```python
from build123d import *

# Parameters (mm, degrees)
SKETCH1_W           = 66.15
SKETCH1_H           = 4
SKETCH1_H_2         = 29.25
SKETCH1_R           = 1.5
BOSS_EXTRUDE1_DEPTH = 4
BOSS_EXTRUDE2_START = 4
SKETCH1_3_W         = 66.15
SKETCH1_3_H         = 4
BOSS_EXTRUDE2_DEPTH = 9
SKETCH2_R           = 1.5
SKETCH2_R_2         = 2.031128953
CUT_EXTRUDE1_DEPTH  = 9


with BuildPart() as part:
    # Sketch1 → Boss-Extrude1 (new body)
    with BuildSketch(Plane(origin=(0, 0, 0), x_dir=(1, 0, 0), z_dir=(0, 1, 0))):
        with Locations((0, -16.625)):
            Rectangle(SKETCH1_W, SKETCH1_H)
        Rectangle(SKETCH1_W, SKETCH1_H_2)
        with Locations((28.075, 9.625)):
            Circle(SKETCH1_R, mode=Mode.SUBTRACT)
        with Locations((28.075, -9.625)):
            Circle(SKETCH1_R, mode=Mode.SUBTRACT)
        with Locations((-28.075, -9.625)):
            Circle(SKETCH1_R, mode=Mode.SUBTRACT)
        with Locations((-28.075, 9.625)):
            Circle(SKETCH1_R, mode=Mode.SUBTRACT)
    extrude(amount=BOSS_EXTRUDE1_DEPTH)

    # Sketch1<3> → Boss-Extrude2 (add)
    with BuildSketch(Plane(origin=(0, 0, 0), x_dir=(1, 0, 0), z_dir=(0, 1, 0)).offset(BOSS_EXTRUDE2_START)):
        with Locations((0, -16.625)):
            Rectangle(SKETCH1_3_W, SKETCH1_3_H)
    extrude(amount=BOSS_EXTRUDE2_DEPTH)

    # Sketch2 → Cut-Extrude1 (cut)
    with BuildSketch(Plane.XY.offset(18.625)):
        with Locations((-24.96, 9)):
            Circle(SKETCH2_R)
        with Locations((24.96, 9)):
            Circle(SKETCH2_R_2)
    extrude(amount=-CUT_EXTRUDE1_DEPTH, mode=Mode.SUBTRACT)


solid = part.part
```
Check sheet for the modelled part. Datum: model origin and axes. Units: mm. A direction names the side the tool comes from. Give positions to 0.01 mm unless a question says otherwise; leave off trailing zeros. Order: outer loops, then holes, each group sorted by start corner. A loop starts at its lowest first (then second) coordinate and runs counter-clockwise, first axis right, second up. Notation, with made-up numbers: (-5.75, 51.5) -> (23.25, 51.5) arc R9 ccw to (23.25, 67.5) -> close; hole circle Ø7 at (71.5, 33). An arc over 180 degrees is marked (long way). Use CSV: the item, a comma, the result in double quotes. Start each with the question number.
1) Material ranges on line 1 (X direction, y = 1.75, z = 11) (3 decimals); line 2 (X direction, y = 1.75, z = -10) (3 decimals); line 3 (Y direction, x = -24.96, z = 17.15), recorded low to high. Write a range as from..to.
2) Set-up check for faces 1 (the face through (0, 8, 14.625)), 2 (the face through (0, 6, 18.625)): record each of +Z, -Z, +X, -X, +Y, -Y from which the full face is reachable in a straight line by a thin tool's end or side.
3) Sectioned sample at A-A, the plane x = 24.96. Record the boundary of the cut face in (y, z) (3 decimals), plus the area to 3 significant figures.
4) Mould release check, pull along Y, two halves, no side actions. Record for faces 3 (the face through (-26.69, 1.97, 10.2)), 4 (the face through (23.46, 10.37, 16.65)), 5 (the face through (0, 0, 2)), 6 (the face through (0, 4, 0)): released by +Y, released by -Y, zero draft, split by the parting line, or undercut.
5) Sectioned sample at C-C, the plane z = -9. Record the boundary of the cut face in (x, y) (3 decimals), plus the area to 3 significant figures.
6) Go/stop test with flat-tipped pins: P1, Ø3, axis at x = -19, z = 7.5, coming from the +Y side; P2, Ø5, axis at y = 8, z = 11, coming from the +X side; P3, Ø2.5, axis at x = -16, y = 7, coming from the -Z side (3 decimals). Record where each tip stops, or that it passes through.
7) Sectioned sample at B-B, the plane y = 9. Record the boundary of the cut face in (x, z) (3 decimals).
8) Sectioned sample at D-D, the plane x = -24.96. Record the boundary of the cut face in (y, z) (3 decimals).
Recorded:
1,line 1,"-33.075..-28.674, -27.476..27.476, 28.674..33.075"
1,line 2,"-33.075..-29.527, -26.623..26.623, 29.527..33.075"
1,line 3,"0..7.5, 10.5..13"
2,face 1,"-Z, +X, -X, +Y"
2,face 2,"+Z, +X, -X, +Y, -Y"
3,outline,"(0, -14.625) -> (4, -14.625) -> (4, 14.625) -> (6.969, 14.625) -> (6.969, 18.625) -> (0, 18.625) -> close; (11.031, 14.625) -> (13, 14.625) -> (13, 18.625) -> (11.031, 18.625) -> close"
3,area,"153 mm2"
4,face 3,"zero draft"
4,face 4,"undercut"
4,face 5,"released by -Y"
4,face 6,"released by +Y"
5,outline,"(-33.075, 0) -> (-29.439, 0) -> (-29.439, 4) -> (-33.075, 4) -> close; (-26.711, 0) -> (26.711, 0) -> (26.711, 4) -> (-26.711, 4) -> close; (29.439, 0) -> (33.075, 0) -> (33.075, 4) -> (29.439, 4) -> close"
5,area,"243 mm2"
6,P1,"y = 4"
6,P2,"through"
6,P3,"z = 14.625"
7,outline,"(-33.075, 14.625) -> (-26.46, 14.625) -> (-26.46, 18.625) -> (-33.075, 18.625) -> close; (-23.46, 14.625) -> (22.929, 14.625) -> (22.929, 18.625) -> (-23.46, 18.625) -> close; (26.991, 14.625) -> (33.075, 14.625) -> (33.075, 18.625) -> (26.991, 18.625) -> close"
8,outline,"(0, -14.625) -> (4, -14.625) -> (4, 14.625) -> (7.5, 14.625) -> (7.5, 18.625) -> (0, 18.625) -> close; (10.5, 14.625) -> (13, 14.625) -> (13, 18.625) -> (10.5, 18.625) -> close"
